Geometry check sheet. Reference: the model listing, model coordinates, mm. Face numbers are marked on the shaded views. Give positions to 0.01 mm unless a question says otherwise; leave off trailing zeros. Loops run counter-clockwise (first coordinate to the right, second up) from the corner with the lowest first, then second, coordinate; pieces in that order, holes last.
1. Go/stop test with flat-tipped pins: pin 1 Ø8 at (x, z) = (-7.5, 9.5) entering from +Y; pin 2 Ø1.1 at (x, y) = (8, 1) entering from +Z. Record where each tip stops, or that it passes through.
2. Material ranges on L1, parallel to X at y = 0.6, z = 13; L2, parallel to X at y = 1.1, z = -13.5; L3, parallel to Y at x = -42, z = 12.5, recorded low to high.
3. Release check for a two-part mould opening along X. For the marked faces 1 and 2 record: +X half, -X half, draft (parallel to the pull), parting line (faces both ways), or undercut.
4. Cross-section at C-C, the plane z = -17. Record the cut outline in (x, y), plus the area to 3 significant figures.
5. Cross-section at A-A, the plane x = 9.5. Record the cut outline in (y, z).
6. Cross-section at B-B, the plane y = 1.25. Record the cut outline in (x, z), plus the area to 3 significant figures.
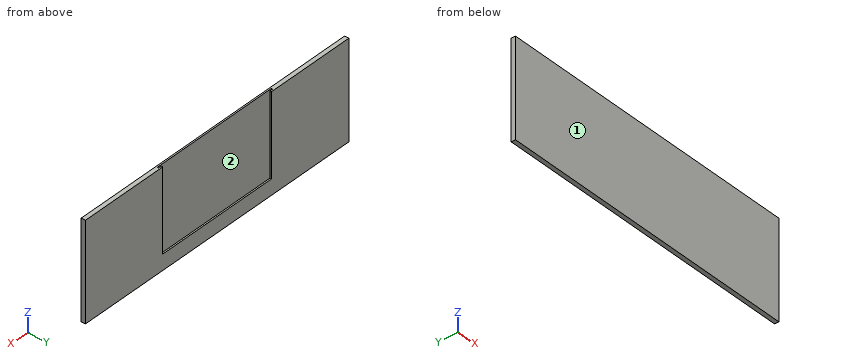
from build123d import *

# Parameters (mm, degrees)
SKETCH1_W           = 87.5
SKETCH1_H           = 57.7
BOSS_EXTRUDE1_DEPTH = 1
BOSS_EXTRUDE2_DEPTH = 1.816115501
BOSS_EXTRUDE3_DEPTH = 1


with BuildPart() as part:
    # Sketch1 → Boss-Extrude1 (new body)
    with BuildSketch(Plane(origin=(0, 0, 0), x_dir=(1, 0, 0), z_dir=(0, 1, 0))):
        Polygon((-101, -33.1), (-45.75, -33.1), (-45.75, 26.6), (45.75, 26.6), (45.75, -33.1), (101, -33.1), (101, 33.1), (-101, 33.1), align=None)
        with Locations((0, -4.25)):
            Rectangle(SKETCH1_W, SKETCH1_H)
        Polygon((-45.75, 26.6), (-45.75, -33.1), (-43.75, -33.1), (-43.75, 24.6), (43.75, 24.6), (43.75, -33.1), (45.75, -33.1), (45.75, 26.6), align=None)
    extrude(amount=-BOSS_EXTRUDE1_DEPTH)

    # Sketch1_3 → Boss-Extrude2 (add)
    with BuildSketch(Plane(origin=(0, 0, 0), x_dir=(1, 0, 0), z_dir=(0, 1, 0))):
        Polygon((-101, -33.1), (-45.75, -33.1), (-45.75, 26.6), (45.75, 26.6), (45.75, -33.1), (101, -33.1), (101, 33.1), (-101, 33.1), align=None)
        Polygon((-45.75, 26.6), (-45.75, -33.1), (-43.75, -33.1), (-43.75, 24.6), (43.75, 24.6), (43.75, -33.1), (45.75, -33.1), (45.75, 26.6), align=None)
    extrude(amount=BOSS_EXTRUDE2_DEPTH)

    # Sketch2 → Boss-Extrude3 (add)
    with BuildSketch(Plane(origin=(0, 1.816115501, 0), x_dir=(1, 0, 0), z_dir=(0, 1, 0))):
        Polygon((-43.75, -33.1), (-41.75, -33.1), (-41.75, 22.6), (41.75, 22.6), (41.75, -33.1), (43.75, -33.1), (43.75, 24.6), (-43.75, 24.6), align=None)
    extrude(amount=-BOSS_EXTRUDE3_DEPTH)


solid = part.part
Result:
1. pin 1: stops at y = 0
1. pin 2: stops at z = -22.6
2. L1: x = -101 to -43.75, 43.75 to 101
2. L2: x = -101 to -41.75, 41.75 to 101
2. L3: y = -1 to 0, 0.82 to 1.82
3. face 1: draft
3. face 2: undercut
4. outline: (-101, -1) - (101, -1) - (101, 1.82) - (41.75, 1.82) - (41.75, 0.82) - (43.75, 0.82) - (43.75, 0) - (-43.75, 0) - (-43.75, 0.82) - (-41.75, 0.82) - (-41.75, 1.82) - (-101, 1.82) - close
4. area: 414 mm2
5. outline: (-1, -33.1) - (1.82, -33.1) - (1.82, -22.6) - (0.82, -22.6) - (0.82, -24.6) - (0, -24.6) - (0, 33.1) - (-1, 33.1) - close
6. outline: (-101, -33.1) - (101, -33.1) - (101, 33.1) - (41.75, 33.1) - (41.75, -22.6) - (-41.75, -22.6) - (-41.75, 33.1) - (-101, 33.1) - close
6. area: 8,720 mm2
